Build history of the part. All positions in model axes, mm. Give positions to 0.01 mm unless a question says otherwise; leave off trailing zeros. Loops run counter-clockwise (first coordinate to the right, second up) from the corner with the lowest first, then second, coordinate; pieces in that order, holes last. Notation, with made-up numbers: M 25.25,-13 L 30.25,-13 A14 cw 30.25,1 Z; hole C -6.75,-40 d3. An arc over 180 degrees is marked long. Answer in a Markdown table with one row per item. Add a question column.
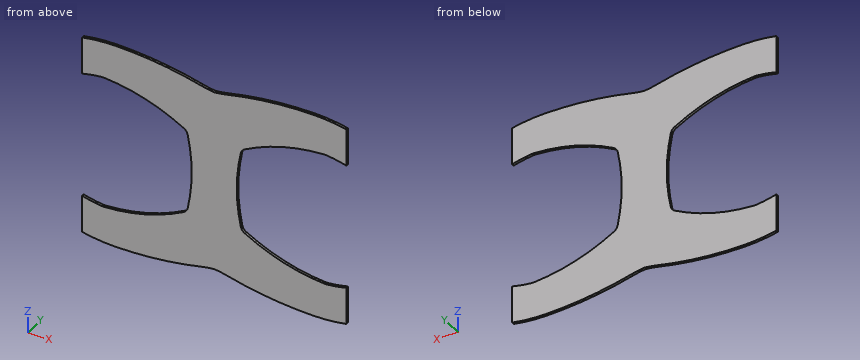
```python
from build123d import *

# Parameters (mm, degrees)
BOSS_EXTRUDE1_START = -10
BOSS_EXTRUDE1_DEPTH = 3


with BuildPart() as part:
    # Sketch1 → Boss-Extrude1 (new body)
    with BuildSketch(Plane(origin=(0, 0, 0), x_dir=(1, 0, 0), z_dir=(0, 1, 0)).offset(BOSS_EXTRUDE1_START)):
        with BuildLine():
            Line((319, 246), (319, 201))
            ThreePointArc((319, 201), (307.388484736, 203.573435825), (295.616405389, 205.2669548))
            ThreePointArc((295.616405389, 205.2669548), (294.01464809, 205.37142016), (292.409672101, 205.347098762))
            ThreePointArc((292.409672101, 205.347098762), (242.780979678, 196.828732334), (196.389162845, 177.248921069))
            ThreePointArc((196.389162845, 177.248921069), (193.242585284, 174.455386906), (191.523683958, 170.614792982))
            ThreePointArc((191.523683958, 170.614792982), (186.742852856, 125), (191.523683958, 79.385207018))
            ThreePointArc((191.523683958, 79.385207018), (193.242585284, 75.544613094), (196.389162845, 72.751078931))
            ThreePointArc((196.389162845, 72.751078931), (242.780979678, 53.171267666), (292.409672101, 44.652901238))
            ThreePointArc((292.409672101, 44.652901238), (294.01464809, 44.62857984), (295.616405389, 44.7330452))
            ThreePointArc((295.616405389, 44.7330452), (307.388484736, 46.426564175), (319, 49))
            Line((319, 49), (319, 4))
            ThreePointArc((319, 4), (299.099751242, 1.002487578), (279, 0))
            ThreePointArc((279, 0), (226.377523813, 3.136099081), (174.5, 12.5))
            ThreePointArc((174.5, 12.5), (167.04561677, 14.023700621), (159.5, 15))
            ThreePointArc((159.5, 15), (151.95438323, 14.023700621), (144.5, 12.5))
            ThreePointArc((144.5, 12.5), (92.622476187, 3.136099081), (40, 0))
            ThreePointArc((40, 0), (19.900248758, 1.002487578), (0, 4))
            Line((0, 4), (0, 49))
            ThreePointArc((0, 49), (11.611515264, 46.426564175), (23.383594611, 44.7330452))
            ThreePointArc((23.383594611, 44.7330452), (24.98535191, 44.62857984), (26.590327899, 44.652901238))
            ThreePointArc((26.590327899, 44.652901238), (76.219020322, 53.171267666), (122.610837155, 72.751078931))
            ThreePointArc((122.610837155, 72.751078931), (125.757414716, 75.544613094), (127.476316042, 79.385207018))
            ThreePointArc((127.476316042, 79.385207018), (132.257147144, 125), (127.476316042, 170.614792982))
            ThreePointArc((127.476316042, 170.614792982), (125.757414716, 174.455386906), (122.610837155, 177.248921069))
            ThreePointArc((122.610837155, 177.248921069), (76.219020322, 196.828732334), (26.590327899, 205.347098762))
            ThreePointArc((26.590327899, 205.347098762), (24.98535191, 205.37142016), (23.383594611, 205.2669548))
            ThreePointArc((23.383594611, 205.2669548), (11.611515264, 203.573435825), (0, 201))
            Line((0, 201), (0, 246))
            ThreePointArc((0, 246), (19.900248758, 248.997512422), (40, 250))
            ThreePointArc((40, 250), (92.622476187, 246.863900919), (144.5, 237.5))
            ThreePointArc((144.5, 237.5), (151.95438323, 235.976299379), (159.5, 235))
            ThreePointArc((159.5, 235), (167.04561677, 235.976299379), (174.5, 237.5))
            ThreePointArc((174.5, 237.5), (226.377523813, 246.863900919), (279, 250))
            ThreePointArc((279, 250), (299.099751242, 248.997512422), (319, 246))
        make_face()
    extrude(amount=-BOSS_EXTRUDE1_DEPTH)


solid = part.part
```
(1) Slice it at D-D, the plane z = -118.5. Give the cut face in (x, y).
(2) Slice it at B-B, the plane x = 97. Give the cut face in (y, z), then the cut area to 3 significant figures.
(3) Slice it at C-C, the plane x = 31. Give the cut face in (y, z).
(4) Wall check: line 1 (X direction, y = -10.55, z = -127.5); line 2 (Z direction, x = 66, y = -11.45); line 3 (Z direction, x = 253.5, y = -11.55). Give the ranges that are in metal, low to high.
Solution:
| question | item | result |
|---|---|---|
| 1 | outline | M 132.16,-13 L 186.84,-13 L 186.84,-10 L 132.16,-10 Z |
| 2 | outline | M -13,-246.32 L -10,-246.32 L -10,-189.6 L -13,-189.6 Z; M -13,-60.4 L -10,-60.4 L -10,-3.68 L -13,-3.68 Z |
| 2 | area | 340 mm^2 |
| 3 | outline | M -13,-249.8 L -10,-249.8 L -10,-205.06 L -13,-205.06 Z; M -13,-44.94 L -10,-44.94 L -10,-0.2 L -13,-0.2 Z |
| 4 | line 1 | 132.24 to 186.76 |
| 4 | line 2 | -249.24 to -199.55, -50.45 to -0.76 |
| 4 | line 3 | -249.27 to -199.67, -50.33 to -0.73 |
